For this review, take the finished solid that the model builds, in its own axes (mm). Coordinates: 2 decimals unless noted, no trailing zeros. Order: outer loops, then holes, each group sorted by start corner. A loop starts at its lowest first (then second) coordinate and runs counter-clockwise, first axis right, second up. Notation, with made-up numbers: (-17.5, 32) -> (25.5, 32) arc R16 ccw to (25.5, 59) -> close; hole circle Ø4 at (17, 18.5). An arc over 180 degrees is marked (long way). Return JSON: item names as keys, results as strings. Group by question number.
Item 1: Insertion check: pin 1 (5 mm diameter, centred on x = 60, y = 105.2, fed in from +Z); pin 2 (1.8 mm diameter, centred on x = -60, y = 25.2, fed in from -Z). Each pin has a flat end and moves straight along its axis. Give the tip position at first contact, or say it passes through.
Item 2: For line 1 along X through (y, z) = (105.2, 0.65); line 2 along Y through (x, z) = (60, 1.55); line 3 along Y through (x, z) = (44, 0.8), list the stretches that pass through material, from the lowest coordinate up.
Item 3: Take a section at A-A (x = -44). Write out the cut boundary in (y, z), then the cut area to 3 significant figures.
Item 4: Draft analysis for pull direction X (two halves, no side actions). For faces 1 (the flat face through (-1, 0, 1)), 2 (the cylindrical face through (61.43, 25.65, 1.48)), 3 (the flat face through (72.5, 64, 1)), state which applies: +X half, -X half, draft (parallel to the pull), parting line (faces both ways), or undercut.
```python
from build123d import *

# Parameters (mm, degrees)
SKETCH1_W             = 145
SKETCH1_H             = 130.4
SKETCH1_R             = 1.5
BOSS_EXTRUDE1_DEPTH   = 3
SKETCH3_R             = 1.7
DEPENDENT_HOLES_DEPTH = 10


with BuildPart() as part:
    # Sketch1 → Boss-Extrude1 (new body)
    with BuildSketch(Plane.XY):
        with Locations((0, 65.2)):
            Rectangle(SKETCH1_W, SKETCH1_H)
        with Locations((-60, 105.2)):
            Circle(SKETCH1_R, mode=Mode.SUBTRACT)
        with Locations((60, 105.2)):
            Circle(SKETCH1_R, mode=Mode.SUBTRACT)
        with Locations((60, 25.2)):
            Circle(SKETCH1_R, mode=Mode.SUBTRACT)
        with Locations((-60, 25.2)):
            Circle(SKETCH1_R, mode=Mode.SUBTRACT)
    extrude(amount=BOSS_EXTRUDE1_DEPTH)

    # Sketch3 → dependent_holes (cut)
    with BuildSketch(Plane.XY.offset(3)):
        with Locations((-57.5, 124.4)):
            Circle(SKETCH3_R)
        with Locations((57.5, 124.4)):
            Circle(SKETCH3_R)
        with Locations((-44, 63.438804225)):
            Circle(SKETCH3_R)
        with Locations((-44, 23.438804225)):
            Circle(SKETCH3_R)
        with Locations((44, 23.438804225)):
            Circle(SKETCH3_R)
        with Locations((44, 63.438804225)):
            Circle(SKETCH3_R)
        with Locations((-34.9875, 6.5)):
            Circle(SKETCH3_R)
        with Locations((34.9875, 6.5)):
            Circle(SKETCH3_R)
    extrude(amount=-DEPENDENT_HOLES_DEPTH, mode=Mode.SUBTRACT)


solid = part.part
```
Findings below:
{
 "1": {"pin 1": "stops at z = 3", "pin 2": "passes through"},
 "2": {"line 1": "x = -72.5 to -61.5, -58.5 to 58.5, 61.5 to 72.5", "line 2": "y = 0 to 23.7, 26.7 to 103.7, 106.7 to 130.4", "line 3": "y = 0 to 21.74, 25.14 to 61.74, 65.14 to 130.4"},
 "3": {"outline": "(0, 0) -> (21.74, 0) -> (21.74, 3) -> (0, 3) -> close; (25.14, 0) -> (61.74, 0) -> (61.74, 3) -> (25.14, 3) -> close; (65.14, 0) -> (130.4, 0) -> (130.4, 3) -> (65.14, 3) -> close", "area": "371 mm2"},
 "4": {"face 1": "draft", "face 2": "undercut", "face 3": "+X half"}
}
